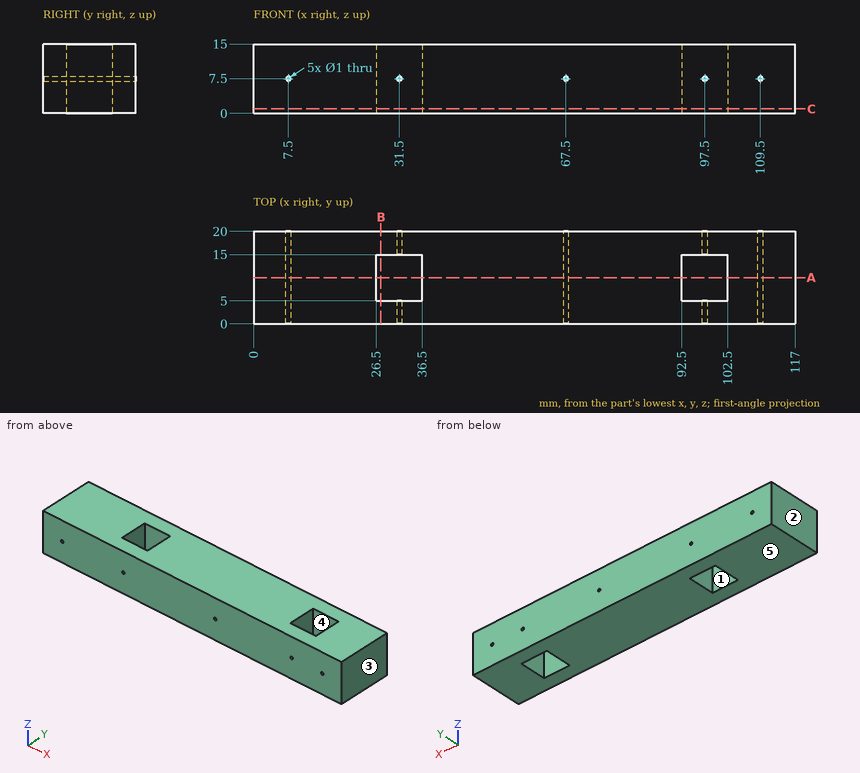
Check sheet for the drawn part. Datum: minimum x, y, z corner. Units: mm. A direction names the side the tool comes from. Round coordinates to 2 decimals unless told otherwise and drop trailing zeros. Order: outer loops, then holes, each group sorted by start corner. A loop starts at its lowest first (then second) coordinate and runs counter-clockwise, first axis right, second up. Notation, with made-up numbers: (89.25, 75.5) -> (136.25, 75.5) arc R26 cw to (136.25, 95.5) -> close; hole circle Ø3 at (-37, 31.25). An arc over 180 degrees is marked (long way). Put each result on its own line as item: value. Start each with the question number.
(1) Depth check by flat-ended pin: pin 1 Ø10 at (x, y) = (100, 6) entering from -Z. Enter the tip coordinate at first touch or a pass-through.
(2) Tool access check on the marked faces 4 and 5. Record the directions out of +Z, -Z, +X, -X, +Y, -Y that give a thin tool (end or side, any length) a straight path to the whole face; none if there is none.
(3) Section check A-A (y = 10). Enter the section's corners in (x, z), then the cut area to 3 significant figures.
(4) Draft check along X on the marked faces 1, 2 and 3. Enter one of: +X half, -X half, draft (parallel to the pull), parting line (faces both ways), or undercut.
(5) Section check C-C (z = 1). Enter the section's corners in (x, y), then the cut area to 3 significant figures.
(6) Material ranges on line 1 along X through (y, z) = (9.5, 13); line 2 along Y through (x, z) = (33, 13.5); line 3 along Z through (x, y) = (31.5, 16.35), recorded low to high.
(7) Section check B-B (x = 27.5). Enter the section's corners in (y, z).
Completed:
1. pin 1: stops at z = 0
2. face 4: +Z, -Z
2. face 5: -Z, +X, -X, +Y, -Y
3. outline: (0, 0) -> (26.5, 0) -> (26.5, 15) -> (0, 15) -> close; (36.5, 0) -> (92.5, 0) -> (92.5, 15) -> (36.5, 15) -> close; (102.5, 0) -> (117, 0) -> (117, 15) -> (102.5, 15) -> close; hole circle Ø1 at (7.5, 7.5); hole circle Ø1 at (67.5, 7.5); hole circle Ø1 at (109.5, 7.5)
3. area: 1,450 mm2
4. face 1: undercut
4. face 2: -X half
4. face 3: +X half
5. outline: (0, 0) -> (117, 0) -> (117, 20) -> (0, 20) -> close; hole (26.5, 5) -> (36.5, 5) -> (36.5, 15) -> (26.5, 15) -> close; hole (92.5, 5) -> (102.5, 5) -> (102.5, 15) -> (92.5, 15) -> close
5. area: 2,140 mm2
6. line 1: x = 0 to 26.5, 36.5 to 92.5, 102.5 to 117
6. line 2: y = 0 to 5, 15 to 20
6. line 3: z = 0 to 7, 8 to 15
7. outline: (0, 0) -> (5, 0) -> (5, 15) -> (0, 15) -> close; (15, 0) -> (20, 0) -> (20, 15) -> (15, 15) -> close
